CAD build for the part. Positions are in the model's coordinates, mm. A direction names the side the tool comes from. Give positions to 0.01 mm unless a question says otherwise; leave off trailing zeros. Write each loop counter-clockwise with the first axis right and the second up, starting at its lowest first coordinate (ties: lowest second). Pieces come first, ordered by that corner, then holes. Notation, with made-up numbers: (56, -1) - (90, -1) arc R13 cw to (90, 17) - close; hole circle Ø10 at (70, 60). An arc over 180 degrees is marked (long way). Answer as a JSON object with one key per item and string values.
from build123d import *

# Parameters (mm, degrees)
BOSS_EXTRUDE2_DEPTH = 30
SKETCH5_R           = 2.5
CUT_EXTRUDE3_DEPTH  = 6
SKETCH6_R           = 2.5
CUT_EXTRUDE4_DEPTH  = 6
BOSS_EXTRUDE3_DEPTH = 5
BOSS_EXTRUDE4_DEPTH = 5
FILLET1_R           = 3
FILLET2_R           = 3
FILLET3_R           = 3
CUT_EXTRUDE5_DEPTH  = 118.046999107
SKETCH10_R          = 3
CUT_EXTRUDE6_DEPTH  = 118.04699927


with BuildPart() as part:
    # Sketch4 → Boss-Extrude2 (new body)
    with BuildSketch(Plane.XY):
        Polygon((0, 0), (0, 80), (5, 80), (5, 5), (80, 5), (80, 0), align=None)
    extrude(amount=BOSS_EXTRUDE2_DEPTH)

    # Sketch5 → Cut-Extrude3 (cut)
    with BuildSketch(Plane(origin=(0, 5, 0), x_dir=(1, 0, 0), z_dir=(0, 1, 0))):
        with Locations(Location((60, -15, 0), (0, 0, 270))):
            Circle(SKETCH5_R)
        with Locations(Location((40, -15, 0), (0, 0, 270))):
            Circle(SKETCH5_R)
    extrude(amount=-CUT_EXTRUDE3_DEPTH, mode=Mode.SUBTRACT)

    # Sketch6 → Cut-Extrude4 (cut)
    with BuildSketch(Plane(origin=(5, 0, 0), x_dir=(0, 0, -1), z_dir=(1, 0, 0))):
        with Locations(Location((-15, 60, 0), (0, 0, 90))):
            Circle(SKETCH6_R)
        with Locations(Location((-15, 40, 0), (0, 0, 90))):
            Circle(SKETCH6_R)
    extrude(amount=-CUT_EXTRUDE4_DEPTH, mode=Mode.SUBTRACT)

    # Sketch7 → Boss-Extrude3 (add)
    with BuildSketch(Plane(origin=(0, 0, 0), x_dir=(-1, 0, 0), z_dir=(0, 0, -1))):
        Polygon((-5, 80), (-5, 5), (-80, 5), align=None)
    extrude(amount=-BOSS_EXTRUDE3_DEPTH)

    # Sketch8 → Boss-Extrude4 (add)
    with BuildSketch(Plane.XY.offset(30)):
        Polygon((5, 80), (5, 5), (80, 5), align=None)
    extrude(amount=-BOSS_EXTRUDE4_DEPTH)

    # Fillet1
    fillet1_edges = [part.edges().sort_by_distance(p)[0] for p in [
        (5, 42.5, 25),
    ]]
    fillet(fillet1_edges, radius=FILLET1_R)

    # Fillet2
    fillet2_edges = [part.edges().sort_by_distance(p)[0] for p in [
        (5, 42.5, 5),
    ]]
    fillet(fillet2_edges, radius=FILLET2_R)

    # Fillet3
    fillet3_edges = [part.edges().sort_by_distance(p)[0] for p in [
        (44, 5, 5),
        (5, 5, 15),
        (44, 5, 25),
        (5.878679656, 5, 24.121320344),
        (5.878679656, 5, 5.878679656),
    ]]
    fillet(fillet3_edges, radius=FILLET3_R)

    # Sketch9 → Cut-Extrude5 (cut, through all)
    with BuildSketch(Plane.XY.offset(30)):
        with BuildLine():
            Line((5, 80), (80, 5))
            ThreePointArc((80, 5), (28.499618275, 28.499618275), (5, 80))
        make_face()
    extrude(amount=-CUT_EXTRUDE5_DEPTH, mode=Mode.SUBTRACT)

    # Sketch10 → Cut-Extrude6 (cut, through all)
    with BuildSketch(Plane.XY.offset(30)):
        with Locations((15, 15)):
            Circle(SKETCH10_R)
    extrude(amount=-CUT_EXTRUDE6_DEPTH, mode=Mode.SUBTRACT)


solid = part.part
Item 1: Cut at C-C (z = 10). Give the cut face in (x, y), and give its area (3 significant figures).
Entries:
{"outline": "(0, 0) - (80, 0) - (80, 5) - (8, 5) arc R3 cw to (5, 8) - (5, 80) - (0, 80) - close", "area": "777 mm2"}
Item 2: Which spindle directions (+Z, -Z, +X, -X, +Y, -Y) get a long thin tool onto all of the face, cutting with end or side? Do faces 4 (the flat face through (5, 45, 15)), 5 (the flat face through (2, 80, 15)). Say none if no direction does.
Entries:
{"face 4": "+X, +Y", "face 5": "+Z, -Z, +X, -X, +Y"}
Item 3: Probe line 1 (X direction, y = 1, z = 15); line 2 (Y direction, x = 36.5, z = 14.5). List the from-to ranges inside material, lowest first. Write a range as from..to.
Entries:
{"line 1": "0..37.5, 42.5..57.5, 62.5..80", "line 2": "0..5"}
Item 4: Flat gauge pins, fed straight in: P1, Ø7, axis at y = 58.5, z = 15, coming from the +X side; P2, Ø5.5, axis at x = 15, y = 15, coming from the -Z side; P3, Ø7, axis at x = 31, z = 13, coming from the +Y side; P4, Ø10, axis at x = 35, z = 10.5, coming from the +Y side. Where does each tip first touch, or does it go through?
Entries:
{"P1": "x = 5", "P2": "through", "P3": "y = 5", "P4": "y = 6.34"}
Item 5: Cut at A-A (x = 15). Give the cut face in (y, z), and give its area (3 significant figures).
Entries:
{"outline": "(0, 0) - (12, 0) - (12, 5) - (8, 5) arc R3 cw to (5, 8) - (5, 22) arc R3 cw to (8, 25) - (12, 25) - (12, 30) - (0, 30) - close; (18, 0) - (46.39, 0) - (46.39, 5) - (18, 5) - close; (18, 25) - (46.39, 25) - (46.39, 30) - (18, 30) - close", "area": "508 mm2"}
Item 6: Mould opens along Z. For faces 1 (the flat face through (22, 22, 0)), 2 (the cylindrical face through (44.5, 5.9, 5.86)), 3 (the cylindrical face through (12.6, 13.2, 27.5)) say: +Z half, -Z half, draft (parallel to the pull), parting line (faces both ways), or undercut.
Entries:
{"face 1": "-Z half", "face 2": "undercut", "face 3": "draft"}
Item 7: Cut at D-D (x = 60). Give the cut face in (y, z), and give its area (3 significant figures).
Entries:
{"outline": "(0, 0) - (8.99, 0) - (8.99, 5) - (8, 5) arc R3 cw to (5, 8) - (5, 12.5) - (0, 12.5) - close; (0, 17.5) - (5, 17.5) - (5, 22) arc R3 cw to (8, 25) - (8.99, 25) - (8.99, 30) - (0, 30) - close", "area": "169 mm2"}
